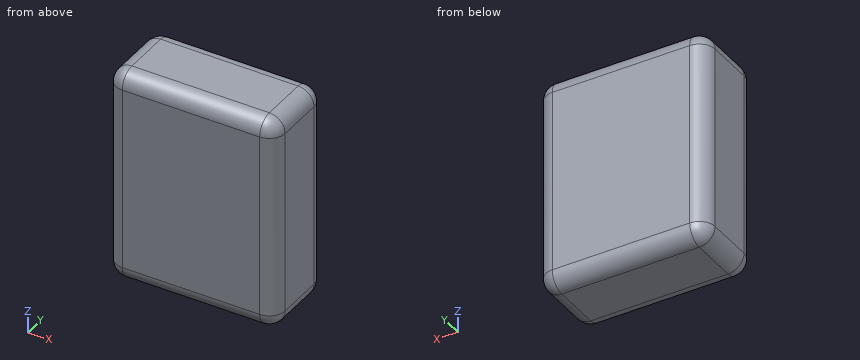
```python
from build123d import *

# Parameters (mm, degrees)
F0_W         = 54.1939660907
F0_H         = 68.9741391689
F1_DEPTH     = 25.4
F2_R         = 5.08
F3_T1_DEPTH  = 58.8141391689
F3_T3_DEPTH  = 44.0339660907
F3_T5_DEPTH  = 15.24
F3_S9_W      = 5.08
F3_S9_H      = 5.08
F3_T10_DEPTH = 5.08
F3_S15_W     = 5.08
F3_S15_H     = 5.08
F3_T16_DEPTH = 5.08
F3_S21_W     = 5.08
F3_S21_H     = 5.08
F3_T22_DEPTH = 5.08
F3_S27_W     = 5.08
F3_S27_H     = 5.08
F3_T28_DEPTH = 5.08
F3_S33_W     = 5.08
F3_S33_H     = 5.08
F3_T34_DEPTH = 5.08
F3_S39_W     = 5.08
F3_S39_H     = 5.08
F3_T40_DEPTH = 5.08
F3_T44_ANGLE = 90
F3_T46_ANGLE = 90


# Not quite as in the source:
# - a fillet or chamfer that OpenCascade refuses, or shapes differently, is made with other operations: its cross-section is extruded or revolved along the edge and cut away or added


with BuildPart() as f1:
    # F0 (on Front) → F1 (new body)
    with BuildSketch(Plane.XZ):
        with Locations((-4.6311207116, -5.9120682999)):
            Rectangle(F0_W, F0_H)
    extrude(amount=F1_DEPTH)

    # F2
    f2_edges = [f1.edges().sort_by_distance(p)[0] for p in [
        (22.465862, -12.7, 28.575001),
        (22.465862, 0, -5.912068),
        (-4.631121, -25.4, 28.575001),
    ]]
    fillet(f2_edges, radius=F2_R)

    # F3: fillet of radius 5.08 on 8 edges, made by hand

    # F3_s2 → F3_t1 (cut)
    with BuildSketch(Plane.XY.offset(-35.3191378844)):
        with BuildLine():
            ThreePointArc((17.3858623338, -25.4), (20.9779647822, -23.9121024484), (22.4658623338, -20.32))
            Line((22.4658623338, -20.32), (22.4658623338, -25.4))
            Line((22.4658623338, -25.4), (17.3858623338, -25.4))
        make_face()
        with BuildLine():
            ThreePointArc((-31.7281037569, -5.08), (-30.2402062053, -1.4878975516), (-26.6481037569, 0))
            Line((-26.6481037569, 0), (-31.7281037569, 0))
            Line((-31.7281037569, 0), (-31.7281037569, -5.08))
        make_face()
        with BuildLine():
            ThreePointArc((-31.7281037569, -20.32), (-30.2402062053, -23.9121024484), (-26.6481037569, -25.4))
            Line((-26.6481037569, -25.4), (-31.7281037569, -25.4))
            Line((-31.7281037569, -25.4), (-31.7281037569, -20.32))
        make_face()
    extrude(amount=F3_T1_DEPTH, mode=Mode.SUBTRACT)

    # F3_s4 → F3_t3 (cut)
    with BuildSketch(Plane.YZ.offset(-26.6481037569)):
        with BuildLine():
            ThreePointArc((-5.08, 28.5750012845), (-1.4878975516, 27.0871037329), (0, 23.4950012845))
            Line((0, 23.4950012845), (0, 28.5750012845))
            Line((0, 28.5750012845), (-5.08, 28.5750012845))
        make_face()
        with BuildLine():
            ThreePointArc((-25.4, -35.3191378844), (-23.9121024484, -38.9112403328), (-20.32, -40.3991378844))
            Line((-20.32, -40.3991378844), (-25.4, -40.3991378844))
            Line((-25.4, -40.3991378844), (-25.4, -35.3191378844))
        make_face()
        with BuildLine():
            ThreePointArc((0, -35.3191378844), (-1.4878975516, -38.9112403328), (-5.08, -40.3991378844))
            Line((-5.08, -40.3991378844), (0, -40.3991378844))
            Line((0, -40.3991378844), (0, -35.3191378844))
        make_face()
    extrude(amount=F3_T3_DEPTH, mode=Mode.SUBTRACT)

    # F3_s6 → F3_t5 (cut)
    with BuildSketch(Plane.XZ.offset(5.08)):
        with BuildLine():
            ThreePointArc((-26.6481037569, 28.5750012845), (-30.2402062053, 27.0871037329), (-31.7281037569, 23.4950012845))
            Line((-31.7281037569, 23.4950012845), (-31.7281037569, 28.5750012845))
            Line((-31.7281037569, 28.5750012845), (-26.6481037569, 28.5750012845))
        make_face()
        with BuildLine():
            ThreePointArc((17.3858623338, -40.3991378844), (20.9779647822, -38.9112403328), (22.4658623338, -35.3191378844))
            Line((22.4658623338, -35.3191378844), (22.4658623338, -40.3991378844))
            Line((22.4658623338, -40.3991378844), (17.3858623338, -40.3991378844))
        make_face()
        with BuildLine():
            ThreePointArc((-31.7281037569, -35.3191378844), (-30.2402062053, -38.9112403328), (-26.6481037569, -40.3991378844))
            Line((-26.6481037569, -40.3991378844), (-31.7281037569, -40.3991378844))
            Line((-31.7281037569, -40.3991378844), (-31.7281037569, -35.3191378844))
        make_face()
    extrude(amount=F3_T5_DEPTH, mode=Mode.SUBTRACT)


with BuildPart() as f3_tool8:
    # F3_s9 → F3_t10 (new body)
    with BuildSketch(Plane.XY.offset(23.4950012845)):
        with Locations((19.9258623338, -2.54)):
            Rectangle(F3_S9_W, F3_S9_H)
    extrude(amount=F3_T10_DEPTH)

    # F3_s11 → F3_t12 (revolve, cut)
    with BuildSketch(Plane(origin=(17.3858623338, -5.08, 23.4950012845), x_dir=(-0.7071067812, -0.7071067812, 0), z_dir=(-0.7071067812, 0.7071067812, 0))):
        with BuildLine():
            ThreePointArc((0, -5.08), (5.08, 0), (0, 5.08))
            Line((0, 5.08), (0, -5.08))
        make_face()
    revolve(axis=Axis((17.3858623338, -5.08, 23.4950012845), (0, 0, 1)), mode=Mode.SUBTRACT)


with BuildPart() as f1_1:
    add(f1.part)

    # F3_t7: cut F3_tool8
    add(f3_tool8.part, mode=Mode.SUBTRACT)


with BuildPart() as f3_tool14:
    # F3_s15 → F3_t16 (new body)
    with BuildSketch(Plane.XZ.offset(20.32)):
        with Locations((19.9258623338, 26.0350012845)):
            Rectangle(F3_S15_W, F3_S15_H)
    extrude(amount=F3_T16_DEPTH)

    # F3_s17 → F3_t18 (revolve, cut)
    with BuildSketch(Plane(origin=(17.3858623338, -20.32, 23.4950012845), x_dir=(-0.7071067812, 0, -0.7071067812), z_dir=(-0.7071067812, 0, 0.7071067812))):
        with BuildLine():
            ThreePointArc((0, -5.08), (5.08, 0), (0, 5.08))
            Line((0, 5.08), (0, -5.08))
        make_face()
    revolve(axis=Axis((17.3858623338, -20.32, 23.4950012845), (0, -1, 0)), mode=Mode.SUBTRACT)


with BuildPart() as f1_2:
    add(f1_1.part)

    # F3_t13: cut F3_tool14
    add(f3_tool14.part, mode=Mode.SUBTRACT)


with BuildPart() as f3_tool20:
    # F3_s21 → F3_t22 (new body)
    with BuildSketch(Plane.YZ.offset(17.3858623338)):
        with Locations((-22.86, -37.8591378844)):
            Rectangle(F3_S21_W, F3_S21_H)
    extrude(amount=F3_T22_DEPTH)

    # F3_s23 → F3_t24 (revolve, cut)
    with BuildSketch(Plane(origin=(17.3858623338, -20.32, -35.3191378844), x_dir=(0, 0.7071067812, 0.7071067812), z_dir=(0, 0.7071067812, -0.7071067812))):
        with BuildLine():
            ThreePointArc((0, -5.08), (5.08, 0), (0, 5.08))
            Line((0, 5.08), (0, -5.08))
        make_face()
    revolve(axis=Axis((17.3858623338, -20.32, -35.3191378844), (1, 0, 0)), mode=Mode.SUBTRACT)


with BuildPart() as f1_3:
    add(f1_2.part)

    # F3_t19: cut F3_tool20
    add(f3_tool20.part, mode=Mode.SUBTRACT)


with BuildPart() as f3_tool26:
    # F3_s27 → F3_t28 (new body)
    with BuildSketch(Plane.XY.offset(23.4950012845)):
        with Locations((-29.1881037569, -2.54)):
            Rectangle(F3_S27_W, F3_S27_H)
    extrude(amount=F3_T28_DEPTH)

    # F3_s29 → F3_t30 (revolve, cut)
    with BuildSketch(Plane(origin=(-26.6481037569, -5.08, 23.4950012845), x_dir=(0.7071067812, -0.7071067812, 0), z_dir=(-0.7071067812, -0.7071067812, 0))):
        with BuildLine():
            ThreePointArc((0, -5.08), (5.08, 0), (0, 5.08))
            Line((0, 5.08), (0, -5.08))
        make_face()
    revolve(axis=Axis((-26.6481037569, -5.08, 23.4950012845), (0, 0, 1)), mode=Mode.SUBTRACT)


with BuildPart() as f1_4:
    add(f1_3.part)

    # F3_t25: cut F3_tool26
    add(f3_tool26.part, mode=Mode.SUBTRACT)


with BuildPart() as f3_tool32:
    # F3_s33 → F3_t34 (new body)
    with BuildSketch(Plane.YZ.offset(-26.6481037569)):
        with Locations((-2.54, -37.8591378844)):
            Rectangle(F3_S33_W, F3_S33_H)
    extrude(amount=-F3_T34_DEPTH)

    # F3_s35 → F3_t36 (revolve, cut)
    with BuildSketch(Plane(origin=(-26.6481037569, -5.08, -35.3191378844), x_dir=(0, -0.7071067812, 0.7071067812), z_dir=(0, -0.7071067812, -0.7071067812))):
        with BuildLine():
            ThreePointArc((0, -5.08), (5.08, 0), (0, 5.08))
            Line((0, 5.08), (0, -5.08))
        make_face()
    revolve(axis=Axis((-26.6481037569, -5.08, -35.3191378844), (-1, 0, 0)), mode=Mode.SUBTRACT)


with BuildPart() as f1_5:
    add(f1_4.part)

    # F3_t31: cut F3_tool32
    add(f3_tool32.part, mode=Mode.SUBTRACT)


with BuildPart() as f3_tool38:
    # F3_s39 → F3_t40 (new body)
    with BuildSketch(Plane.YZ.offset(-26.6481037569)):
        with Locations((-22.86, -37.8591378844)):
            Rectangle(F3_S39_W, F3_S39_H)
    extrude(amount=-F3_T40_DEPTH)

    # F3_s41 → F3_t42 (revolve, cut)
    with BuildSketch(Plane(origin=(-26.6481037569, -20.32, -35.3191378844), x_dir=(0, 0.7071067812, 0.7071067812), z_dir=(0, -0.7071067812, 0.7071067812))):
        with BuildLine():
            ThreePointArc((0, -5.08), (5.08, 0), (0, 5.08))
            Line((0, 5.08), (0, -5.08))
        make_face()
    revolve(axis=Axis((-26.6481037569, -20.32, -35.3191378844), (-1, 0, 0)), mode=Mode.SUBTRACT)


with BuildPart() as f1_6:
    add(f1_5.part)

    # F3_t37: cut F3_tool38
    add(f3_tool38.part, mode=Mode.SUBTRACT)

    # F3_s43 → F3_t44 (revolve, cut)
    with BuildSketch(Plane.XZ.offset(5.08)):
        with BuildLine():
            ThreePointArc((17.3858623338, -40.3991378844), (20.9779647822, -38.9112403328), (22.4658623338, -35.3191378844))
            Line((22.4658623338, -35.3191378844), (22.4658623338, -40.3991378844))
            Line((22.4658623338, -40.3991378844), (17.3858623338, -40.3991378844))
        make_face()
    revolve(axis=Axis((17.3858623338, -5.08, -40.3991378844), (0, 0, 1)), revolution_arc=F3_T44_ANGLE, mode=Mode.SUBTRACT)

    # F3_s45 → F3_t46 (revolve, cut)
    with BuildSketch(Plane.XZ.offset(20.32)):
        with BuildLine():
            ThreePointArc((-31.7281037569, 23.4950012845), (-30.2402062053, 27.0871037329), (-26.6481037569, 28.5750012845))
            Line((-26.6481037569, 28.5750012845), (-31.7281037569, 28.5750012845))
            Line((-31.7281037569, 28.5750012845), (-31.7281037569, 23.4950012845))
        make_face()
    revolve(axis=Axis((-31.7281037569, -20.32, 23.4950012845), (1, 0, 0)), revolution_arc=F3_T46_ANGLE, mode=Mode.SUBTRACT)


solid = f1_6.part
```
Geometry: final body of the model. Coordinates: model frame, mm. Round coordinates to 2 decimals unless told otherwise and drop trailing zeros. Order: outer loops, then holes, each group sorted by start corner. A loop starts at its lowest first (then second) coordinate and runs counter-clockwise, first axis right, second up. Notation, with made-up numbers: (-37.75, -31) - (-7.75, -31) arc R22 cw to (-7.75, 3) - close; hole circle Ø9 at (3.25, 78.5). An arc over 180 degrees is marked (long way). Use CSV: the item, a comma, the result in double quotes. Start each with the question number.
Q1. Material intervals for line 1 along X through (y, z) = (-4.75, 11); line 2 along Y through (x, z) = (-27, 6); line 3 along Z through (x, y) = (-4.5, -4.75), sorted ascending. Write a range as from..to.
Q2. First-contact query: pin 1 (2 mm diameter, centred on x = 15.5, y = -22.5, fed in from +Z). Flat tip, straight axial feed; report the tip coordinate or a pass-through.
Q3. Section query A-A (z = 19). Return loops of the section in (x, y).
Q4. Section query B-B (y = -3.25). Return loops of the section in (x, z) (3 decimals), and give its area (3 significant figures).
Result set:
1,line 1,"x = -31.72..22.46"
1,line 2,"y = -25.39..-0.01"
1,line 3,"z = -40.39..28.56"
2,pin 1,"stops at z = 28.44"
3,outline,"(-31.73, -20.32) arc R5.08 ccw to (-26.65, -25.4) - (17.39, -25.4) arc R5.08 ccw to (22.47, -20.32) - (22.47, -5.08) arc R5.08 ccw to (17.39, 0) - (-26.65, 0) arc R5.08 ccw to (-31.73, -5.08) - close"
4,outline,"(-31.387, -35.319) arc R4.739 ccw to (-26.648, -40.058) - (17.386, -40.058) arc R4.739 ccw to (22.125, -35.319) - (22.125, 23.495) arc R4.739 ccw to (17.386, 28.234) - (-26.648, 28.234) arc R4.739 ccw to (-31.387, 23.495) - close"
4,area,"3,640 mm2"
